```python
from build123d import *

# Parameters (mm, degrees)
SKETCH1_W                                  = 170
SKETCH1_H                                  = 150
BOSS_EXTRUDE1_DEPTH                        = 10
BOSS_EXTRUDE2_DEPTH                        = 170
FILLET1_R                                  = 10
SHELL1_T                                   = -2
SKETCH3_W                                  = 115
SKETCH3_H                                  = 90
CUT_EXTRUDE1_DEPTH                         = 2
SKETCH4_W                                  = 119
SKETCH4_H                                  = 94
SKETCH4_W_2                                = 115
SKETCH4_H_2                                = 90
BOSS_EXTRUDE3_DEPTH                        = 10
SKETCH5_W                                  = 119
SKETCH5_H                                  = 94
BOSS_EXTRUDE4_DEPTH                        = 2
SKETCH6_R                                  = 2.5
CUT_EXTRUDE2_DEPTH                         = 2
SKETCH7_R                                  = 6
CUT_EXTRUDE3_DEPTH                         = 2
SKETCH9_W                                  = 10
SKETCH9_H                                  = 15
BOSS_EXTRUDE5_DEPTH                        = 10
SKETCH10_W                                 = 5
SKETCH10_H                                 = 10
CUT_EXTRUDE4_DEPTH                         = 5
MIRROR1_AT_THE_SECOND_PLANE_COPY_1_SKETC_W = 10
MIRROR1_AT_THE_SECOND_PLANE_COPY_1_SKETC_H = 15
MIRROR1_AT_THE_SECOND_PLANE_COPY_1_DEPTH   = 10
MIRROR1_AT_THE_SECOND_PLANE_COPY_2_SKETC_W = 5
MIRROR1_AT_THE_SECOND_PLANE_COPY_2_SKETC_H = 10
MIRROR1_AT_THE_SECOND_PLANE_COPY_2_DEPTH   = 5
FILLET2_R                                  = 2
SKETCH11_R                                 = 1.5
CUT_EXTRUDE5_DEPTH                         = 2


with BuildPart() as part:
    # Sketch1 → Boss-Extrude1 (new body)
    with BuildSketch(Plane(origin=(0, 0, 0), x_dir=(1, 0, 0), z_dir=(0, 1, 0))):
        Rectangle(SKETCH1_W, SKETCH1_H)
    extrude(amount=BOSS_EXTRUDE1_DEPTH)

    # Sketch2 → Boss-Extrude2 (add)
    with BuildSketch(Plane.ZY.offset(85)):
        Polygon((-75, 10), (-75, 50.192378865), (75, 10), align=None)
    extrude(amount=-BOSS_EXTRUDE2_DEPTH)

    # Fillet1
    fillet1_edges = [part.edges().sort_by_distance(p)[0] for p in [
        (0, 50.192378865, -75),
        (-85, 30.096189432, 0),
        (85, 30.096189432, 0),
        (0, 10, 75),
        (85, 5, 75),
        (-85, 5, 75),
        (-85, 25.096189432, -75),
        (85, 25.096189432, -75),
    ]]
    fillet(fillet1_edges, radius=FILLET1_R)

    # Shell1
    shell1_openings = [part.faces().sort_by_distance(p)[0] for p in [
        (0, 0, 0),
    ]]
    offset(amount=SHELL1_T, openings=shell1_openings, kind=Kind.INTERSECTION)

    # Sketch3 → Cut-Extrude1 (cut)
    with BuildSketch(Plane(origin=(0, 28.080127019, 7.524047358), x_dir=(1, 0, 0), z_dir=(0, 0.96592582628907, 0.25881904510251436))):
        with Locations((0, 10)):
            Rectangle(SKETCH3_W, SKETCH3_H)
    extrude(amount=-CUT_EXTRUDE1_DEPTH, mode=Mode.SUBTRACT)

    # Sketch4 → Boss-Extrude3 (add)
    with BuildSketch(Plane(origin=(0, 26.148275366, 7.006409268), x_dir=(1, 0, 0), z_dir=(0, -0.96592582628907, -0.25881904510251436))):
        with Locations((0, -10)):
            Rectangle(SKETCH4_W, SKETCH4_H)
        with Locations((0, -10)):
            Rectangle(SKETCH4_W_2, SKETCH4_H_2, mode=Mode.SUBTRACT)
    extrude(amount=BOSS_EXTRUDE3_DEPTH)

    # Sketch5 → Boss-Extrude4 (add)
    with BuildSketch(Plane(origin=(0, 16.489017103, 4.418218817), x_dir=(1, 0, 0), z_dir=(0, -0.96592582628907, -0.25881904510251436))):
        with Locations((0, -10)):
            Rectangle(SKETCH5_W, SKETCH5_H)
    extrude(amount=BOSS_EXTRUDE4_DEPTH)

    # Sketch6 → Cut-Extrude2 (cut)
    with BuildSketch(Plane(origin=(0, 28.080127019, 7.524047358), x_dir=(1, 0, 0), z_dir=(0, 0.96592582628907, 0.25881904510251436))):
        with Locations(Location((-62.5, 10, 0), (0, 0, 270))):
            Circle(SKETCH6_R)
        with Locations(Location((-62.5, 40, 0), (0, 0, 270))):
            Circle(SKETCH6_R)
        with Locations(Location((-62.5, -20, 0), (0, 0, 270))):
            Circle(SKETCH6_R)
        with Locations(Location((62.5, -20, 0), (0, 0, 270))):
            Circle(SKETCH6_R)
        with Locations(Location((62.5, 40, 0), (0, 0, 270))):
            Circle(SKETCH6_R)
        with Locations(Location((62.5, 10, 0), (0, 0, 270))):
            Circle(SKETCH6_R)
    extrude(amount=-CUT_EXTRUDE2_DEPTH, mode=Mode.SUBTRACT)

    # Sketch7 → Cut-Extrude3 (cut)
    with BuildSketch(Plane(origin=(0, 28.080127019, 7.524047358), x_dir=(1, 0, 0), z_dir=(0, 0.96592582628907, 0.25881904510251436))):
        with Locations(Location((-12.5, -48.59148832, 0), (0, 0, 270))):
            Circle(SKETCH7_R)
        with Locations(Location((12.5, -48.59148832, 0), (0, 0, 270))):
            Circle(SKETCH7_R)
        with Locations(Location((37.5, -48.59148832, 0), (0, 0, 270))):
            Circle(SKETCH7_R)
        with Locations(Location((-37.5, -48.59148832, 0), (0, 0, 270))):
            Circle(SKETCH7_R)
    extrude(amount=-CUT_EXTRUDE3_DEPTH, mode=Mode.SUBTRACT)

    # Sketch9 → Boss-Extrude5 (add)
    with BuildSketch(Plane.XZ):
        with Locations((-78, -47.5)):
            Rectangle(SKETCH9_W, SKETCH9_H)
    boss_extrude5 = extrude(amount=-BOSS_EXTRUDE5_DEPTH)

    # Sketch10 → Cut-Extrude4 (cut)
    with BuildSketch(Plane.XZ):
        with Locations((-78, -47.5)):
            Rectangle(SKETCH10_W, SKETCH10_H)
    cut_extrude4 = extrude(amount=-CUT_EXTRUDE4_DEPTH, mode=Mode.SUBTRACT)

    # Mirror1: Boss-Extrude5, Cut-Extrude4 across plane
    add(boss_extrude5.mirror(Plane(origin=(0, 0, 0), x_dir=(0, 0, 1), z_dir=(1, 0, 0))))
    add(cut_extrude4.mirror(Plane(origin=(0, 0, 0), x_dir=(0, 0, 1), z_dir=(1, 0, 0))), mode=Mode.SUBTRACT)

    # Mirror1 at the second plane: Boss-Extrude5, Cut-Extrude4 across plane
    add(boss_extrude5.mirror(Plane.XY))
    add(cut_extrude4.mirror(Plane.XY), mode=Mode.SUBTRACT)

    # Mirror1 at the second plane copy 1 sketc → Mirror1 at the second plane copy 1 (add)
    with BuildSketch(Plane(origin=(0, 0, 0), x_dir=(-1, 0, 0), z_dir=(0, -1, 0))):
        with Locations((-78, -47.5)):
            Rectangle(MIRROR1_AT_THE_SECOND_PLANE_COPY_1_SKETC_W, MIRROR1_AT_THE_SECOND_PLANE_COPY_1_SKETC_H)
    extrude(amount=-MIRROR1_AT_THE_SECOND_PLANE_COPY_1_DEPTH)

    # Mirror1 at the second plane copy 2 sketc → Mirror1 at the second plane copy 2 (cut)
    with BuildSketch(Plane(origin=(0, 0, 0), x_dir=(-1, 0, 0), z_dir=(0, -1, 0))):
        with Locations((-78, -47.5)):
            Rectangle(MIRROR1_AT_THE_SECOND_PLANE_COPY_2_SKETC_W, MIRROR1_AT_THE_SECOND_PLANE_COPY_2_SKETC_H)
    extrude(amount=-MIRROR1_AT_THE_SECOND_PLANE_COPY_2_DEPTH, mode=Mode.SUBTRACT)

    # Fillet2
    fillet2_edges = [part.edges().sort_by_distance(p)[0] for p in [
        (-73, 5, -40),
        (-73, 5, -55),
        (-73, 5, 40),
        (-73, 5, 55),
        (73, 5, -55),
        (73, 5, -40),
        (73, 5, 55),
        (73, 5, 40),
    ]]
    fillet(fillet2_edges, radius=FILLET2_R)

    # Sketch11 → Cut-Extrude5 (cut)
    with BuildSketch(Plane(origin=(0, 28.080127019, 7.524047358), x_dir=(1, 0, 0), z_dir=(0, 0.96592582628907, 0.25881904510251436))):
        with Locations(Location((-17.5, 63.701463406, 0), (0, 0, 270))):
            Circle(SKETCH11_R)
        with Locations(Location((17.5, 63.701463406, 0), (0, 0, 270))):
            Circle(SKETCH11_R)
        with Locations(Location((-66.25, -10, 0), (0, 0, 270))):
            Circle(SKETCH11_R)
        with Locations(Location((66.25, -10, 0), (0, 0, 270))):
            Circle(SKETCH11_R)
        with Locations(Location((-66.25, 30, 0), (0, 0, 270))):
            Circle(SKETCH11_R)
        with Locations(Location((66.25, 30, 0), (0, 0, 270))):
            Circle(SKETCH11_R)
    extrude(amount=-CUT_EXTRUDE5_DEPTH, mode=Mode.SUBTRACT)


solid = part.part
```
Input: part model. Units: mm. Frame: model coordinates. A direction names the side the tool comes from. Round coordinates to 2 decimals unless told otherwise and drop trailing zeros. Loops run counter-clockwise (first coordinate to the right, second up) from the corner with the lowest first, then second, coordinate; pieces in that order, holes last. Notation, with made-up numbers: M -6.5,75.25 L 2.5,75.25 A18 ccw 2.5,106.25 Z; hole C 78,43 d1. An arc over 180 degrees is marked long. Answer in a Markdown table with one row per item. Add a question column.
1. Contact query for flat-ended pins moving along their axis: pin 1 (4 mm diameter, centred on y = 19.5, z = 10.5, fed in from -X); pin 2 (5 mm diameter, centred on x = 76.5, z = 48.5, fed in from +Y); pin 3 (8 mm diameter, centred on x = -57.5, z = 38.5, fed in from -Y). Output: stop coordinate, or through.
2. Section A-A (x = 51.5). Output: boundary loops of the cut face in (y, z), and give its area (3 significant figures).
3. Set-up query: faces 4 (the face through (-0.8, 13.3, 39.8)), 5 (the face through (80.5, 2, 48)), 6 (the face through (78, 10, 47)), 7 (the face through (81.99, 18.32, -72.15)). Return all of +Z, -Z, +X, -X, +Y, -Y with unobstructed straight access to the full face (end or side cutting, diameter ignored); none if empty.
4. Ray query, probe 1 along X at (y, z) = (20.5, -26); probe 2 along Z at (x, y) = (-67.5, 2); probe 3 along Y at (x, z) = (66.5, -64.5). Return the intervals inside material, ascending.
5. Mould query, pull axis Z, two halves, no side actions, for faces 1 (the face through (-1.05, 18.035, 45.012)), 2 (the face through (1.05, 45.015, -71.189)), 3 (the face through (-1, 18, -73)). Classes: released by +Z, released by -Z, zero draft, split by the parting line, or undercut.
Values follow:
| question | item | result |
|---|---|---|
| 1 | pin 1 | x = -84.99 |
| 1 | pin 2 | y = 17.71 |
| 1 | pin 3 | y = 4.98 |
| 2 | outline | M 0,-75 L 37.16,-75 A10 ccw 46.82,-62.41 L 42.32,-45.6 L 30.72,-48.71 L 7.43,38.23 L 19.02,41.33 L 11.99,67.59 A10 ccw 2.33,75 L 0,75 L 0,73 L 2.33,73 A8 cw 10.05,67.07 L 16.57,42.75 L 4.98,39.64 L 29.31,-51.16 L 40.9,-48.05 L 44.89,-62.93 A8 cw 37.16,-73 L 0,-73 Z |
| 2 | area | 453 mm^2 |
| 3 | face 4 | +Y |
| 3 | face 5 | -Y |
| 3 | face 6 | none |
| 3 | face 7 | -Z, +X, +Y, -Y |
| 4 | probe 1 | -85 to -83, 83 to 85 |
| 4 | probe 2 | -75 to -73, 73 to 75 |
| 4 | probe 3 | 45.14 to 47.15 |
| 5 | face 1 | released by +Z |
| 5 | face 2 | split by the parting line |
| 5 | face 3 | undercut |
